from build123d import *

# Parameters (mm, degrees)
SKETCH1_W           = 254
SKETCH1_H           = 59
BOSS_EXTRUDE1_DEPTH = 3
SKETCH2_W           = 115
SKETCH2_H           = 54
BOSS_EXTRUDE2_DEPTH = 21
SKETCH3_W           = 111
SKETCH3_H           = 50
CUT_EXTRUDE3_DEPTH  = 21
SKETCH4_R           = 7.2
SKETCH4_R_2         = 24.25
CUT_EXTRUDE4_DEPTH  = 3
SKETCH5_W           = 250
SKETCH5_H           = 59
SKETCH5_W_2         = 111
SKETCH5_H_2         = 50
BOSS_EXTRUDE3_DEPTH = 2
SKETCH6_W           = 59
SKETCH6_H           = 3
BOSS_EXTRUDE4_DEPTH = 4
SKETCH7_W           = 258
SKETCH7_H           = 3
BOSS_EXTRUDE5_DEPTH = 4
SKETCH8_W           = 63
SKETCH8_H           = 3
BOSS_EXTRUDE6_DEPTH = 4
SKETCH9_W           = 250
SKETCH9_H           = 2
BOSS_EXTRUDE7_DEPTH = 1


with BuildPart() as part:
    # Sketch1 → Boss-Extrude1 (new body)
    with BuildSketch(Plane(origin=(0, 0, 0), x_dir=(1, 0, 0), z_dir=(0, 1, 0))):
        Rectangle(SKETCH1_W, SKETCH1_H)
    extrude(amount=BOSS_EXTRUDE1_DEPTH)

    # Sketch2 → Boss-Extrude2 (add)
    with BuildSketch(Plane(origin=(0, 3, 0), x_dir=(1, 0, 0), z_dir=(0, 1, 0))):
        Rectangle(SKETCH2_W, SKETCH2_H)
    extrude(amount=BOSS_EXTRUDE2_DEPTH)

    # Sketch3 → Cut-Extrude3 (cut)
    with BuildSketch(Plane.XZ):
        Rectangle(SKETCH3_W, SKETCH3_H)
    extrude(amount=-CUT_EXTRUDE3_DEPTH, mode=Mode.SUBTRACT)

    # Sketch4 → Cut-Extrude4 (cut)
    with BuildSketch(Plane(origin=(0, 24, 0), x_dir=(1, 0, 0), z_dir=(0, 1, 0))):
        with Locations((-42.1, 0)):
            Circle(SKETCH4_R)
        Circle(SKETCH4_R_2)
        with Locations((42.1, 0)):
            Circle(SKETCH4_R)
    extrude(amount=-CUT_EXTRUDE4_DEPTH, mode=Mode.SUBTRACT)

    # Sketch5 → Boss-Extrude3 (add)
    with BuildSketch(Plane.XZ):
        with Locations((0, 2)):
            Rectangle(SKETCH5_W, SKETCH5_H)
        Rectangle(SKETCH5_W_2, SKETCH5_H_2, mode=Mode.SUBTRACT)
    extrude(amount=BOSS_EXTRUDE3_DEPTH)

    # Sketch6 → Boss-Extrude4 (add)
    with BuildSketch(Plane.ZY.offset(127)):
        with Locations((0, 1.5)):
            Rectangle(SKETCH6_W, SKETCH6_H)
    extrude(amount=BOSS_EXTRUDE4_DEPTH)

    # Sketch7 → Boss-Extrude5 (add)
    with BuildSketch(Plane(origin=(0, 0, -29.5), x_dir=(-1, 0, 0), z_dir=(0, 0, -1))):
        with Locations((2, 1.5)):
            Rectangle(SKETCH7_W, SKETCH7_H)
    extrude(amount=BOSS_EXTRUDE5_DEPTH)

    # Sketch8 → Boss-Extrude6 (add)
    with BuildSketch(Plane(origin=(127, 0, 0), x_dir=(0, 0, -1), z_dir=(1, 0, 0))):
        with Locations((2, 1.5)):
            Rectangle(SKETCH8_W, SKETCH8_H)
    extrude(amount=BOSS_EXTRUDE6_DEPTH)

    # Sketch9 → Boss-Extrude7 (add)
    with BuildSketch(Plane.XY.offset(31.5)):
        with Locations((0, -1)):
            Rectangle(SKETCH9_W, SKETCH9_H)
    extrude(amount=BOSS_EXTRUDE7_DEPTH)


solid = part.part
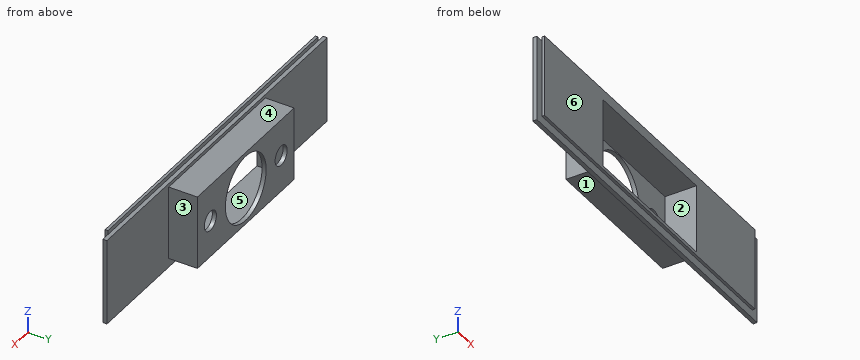
Check sheet for the modelled part. Datum: model origin and axes. Units: mm. Face numbers are marked on the shaded views. A direction names the side the tool comes from. Round coordinates to 2 decimals unless told otherwise and drop trailing zeros. Write each loop counter-clockwise with the first axis right and the second up, starting at its lowest first coordinate (ties: lowest second). Pieces come first, ordered by that corner, then holes. Notation, with made-up numbers: (4.5, 58.25) -> (21.5, 58.25) arc R20 cw to (21.5, 87.25) -> close; hole circle Ø9 at (73.25, -35). An arc over 180 degrees is marked (long way). Answer as CSV lines item,"result". Start each with the question number.
1) Go/stop test with flat-tipped pins: P1, Ø6.5, axis at y = 17.5, z = 4, coming from the +X side; P2, Ø1.6, axis at y = -1.5, z = 0, coming from the +X side; P3, Ø8.5, axis at x = -42.1, z = 0, coming from the +Y side; P4, Ø1, axis at y = 7.5, z = 0.5, coming from the -X side. Record where each tip stops, or that it passes through.
2) Material ranges on line 1 (X direction, y = 23.15, z = 0); line 2 (X direction, y = 17.5, z = -8.5); line 3 (Z direction, x = 1, y = 1.5), recorded low to high. Write a range as from..to.
3) Section check A-A on x = -42.1. Enter the section's corners in (y, z).
4) Section check D-D on x = -88. Enter the section's corners in (y, z), and give its area (3 significant figures).
5) Release check for a two-part mould opening along X. For the marked faces 1, 2 and 3 record: pulls with the +X half, pulls with the -X half, needs draft (parallel to the pull), parting line crosses it, or undercut.
6) Section check B-B on z = 0. Enter the section's corners in (x, y), and give its area (3 significant figures).
7) Tool access check on the marked faces 4, 5 and 6. Record the directions out of +Z, -Z, +X, -X, +Y, -Y that give a thin tool (end or side, any length) a straight path to the whole face; none if there is none.
8) Section check C-C on y = 9.5. Enter the section's corners in (x, z), and give its area (3 significant figures).
Found:
1,P1,"stops at x = 57.5"
1,P2,"stops at x = 125"
1,P3,"passes through"
1,P4,"stops at x = -57.5"
2,line 1,"x = -57.5..-49.3, -34.9..-24.25, 24.25..34.9, 49.3..57.5"
2,line 2,"x = -57.5..-55.5, 55.5..57.5"
2,line 3,"z = -33.5..-25, 25..29.5"
3,outline,"(-2, -27.5) -> (0, -27.5) -> (0, -33.5) -> (3, -33.5) -> (3, -27) -> (24, -27) -> (24, -7.2) -> (21, -7.2) -> (21, -25) -> (-2, -25) -> close; (-2, 25) -> (21, 25) -> (21, 7.2) -> (24, 7.2) -> (24, 27) -> (3, 27) -> (3, 29.5) -> (0, 29.5) -> (0, 32.5) -> (-2, 32.5) -> close"
4,outline,"(-2, -27.5) -> (0, -27.5) -> (0, -33.5) -> (3, -33.5) -> (3, 29.5) -> (0, 29.5) -> (0, 32.5) -> (-2, 32.5) -> close"
4,area,"309 mm^2"
5,face 1,"needs draft"
5,face 2,"undercut"
5,face 3,"pulls with the +X half"
6,outline,"(-131, 0) -> (-125, 0) -> (-125, -2) -> (-55.5, -2) -> (-55.5, 21) -> (-49.3, 21) -> (-49.3, 24) -> (-57.5, 24) -> (-57.5, 3) -> (-131, 3) -> close; (-34.9, 21) -> (-24.25, 21) -> (-24.25, 24) -> (-34.9, 24) -> close; (24.25, 21) -> (34.9, 21) -> (34.9, 24) -> (24.25, 24) -> close; (49.3, 21) -> (55.5, 21) -> (55.5, -2) -> (125, -2) -> (125, 0) -> (131, 0) -> (131, 3) -> (57.5, 3) -> (57.5, 24) -> (49.3, 24) -> close"
6,area,"916 mm^2"
7,face 4,"+Z, +X, -X, +Y"
7,face 5,"-Y"
7,face 6,"+Z, -Z, +X, -X, -Y"
8,outline,"(-57.5, -27) -> (57.5, -27) -> (57.5, 27) -> (-57.5, 27) -> close; hole (-55.5, -25) -> (55.5, -25) -> (55.5, 25) -> (-55.5, 25) -> close"
8,area,"660 mm^2"
